from build123d import *

# Parameters (mm, degrees)
BOX697_W                     = 6
BOX697_H                     = 6
BOX697_DEPTH                 = 2
BOX697_PLACEMENT_ANGLE       = 45
BOX703_W                     = 6
BOX703_H                     = 6
BOX703_DEPTH                 = 2
BOX703_PLACEMENT_ANGLE       = 45
BOX702_W                     = 6
BOX702_H                     = 6
BOX702_DEPTH                 = 2
BOX701_W                     = 6
BOX701_H                     = 6
BOX701_DEPTH                 = 2
BOX701_PLACEMENT_ANGLE       = 225
BOX700_W                     = 6
BOX700_H                     = 6
BOX700_DEPTH                 = 2
BOX699_W                     = 6
BOX699_H                     = 6
BOX699_DEPTH                 = 2
BOX699_PLACEMENT_ANGLE       = 135
BOX698_W                     = 6
BOX698_H                     = 6
BOX698_DEPTH                 = 2
BOX696_W                     = 6
BOX696_H                     = 6
BOX696_DEPTH                 = 2
CYLINDER1770_R               = 1.5
CYLINDER1770_DEPTH           = 30
CYLINDER1770_PLACEMENT_ANGLE = 45
CYLINDER1768_R               = 1.5
CYLINDER1768_DEPTH           = 30
CYLINDER1764_R               = 1.5
CYLINDER1764_DEPTH           = 30
CYLINDER1764_PLACEMENT_ANGLE = 135
CYLINDER1767_R               = 1.5
CYLINDER1767_DEPTH           = 30
CYLINDER1765_R               = 1.5
CYLINDER1765_DEPTH           = 30
CYLINDER1765_PLACEMENT_ANGLE = 225
CYLINDER1769_R               = 1.5
CYLINDER1769_DEPTH           = 30
CYLINDER1766_R               = 1.5
CYLINDER1766_DEPTH           = 30
CYLINDER1766_PLACEMENT_ANGLE = 45
CYLINDER1771_R               = 1.5
CYLINDER1771_DEPTH           = 30
TUBE086_R                    = 35
TUBE086_R_2                  = 29.1
TUBE086_DEPTH                = 16


with BuildPart() as krychle697:
    # Box697 → Box697 (new body)
    with BuildSketch(Plane.XY):
        with Locations((3, 3)):
            Rectangle(BOX697_W, BOX697_H)
    extrude(amount=BOX697_DEPTH)


with BuildPart() as krychle697_1:
    # Box697 placement: moved
    add(krychle697.part.moved(Location((22.627417, -26.870058, 6))).rotate(Axis((22.627417, -26.870058, 6), (0, 0, 1)), BOX697_PLACEMENT_ANGLE))


with BuildPart() as krychle703:
    # Box703 → Box703 (new body)
    with BuildSketch(Plane.XY):
        with Locations((3, 3)):
            Rectangle(BOX703_W, BOX703_H)
    extrude(amount=BOX703_DEPTH)


with BuildPart() as krychle703_1:
    # Box703 placement: moved
    add(krychle703.part.moved(Location((-26.870058, -22.627417, 6))).rotate(Axis((-26.870058, -22.627417, 6), (0, 0, -1)), BOX703_PLACEMENT_ANGLE))


with BuildPart() as krychle702:
    # Box702 → Box702 (new body)
    with BuildSketch(Plane(origin=(-35, 3, 6), x_dir=(0, -1, 0), z_dir=(0, 0, 1))):
        with Locations((3, 3)):
            Rectangle(BOX702_W, BOX702_H)
    extrude(amount=BOX702_DEPTH)


with BuildPart() as krychle701:
    # Box701 → Box701 (new body)
    with BuildSketch(Plane.XY):
        with Locations((3, 3)):
            Rectangle(BOX701_W, BOX701_H)
    extrude(amount=BOX701_DEPTH)


with BuildPart() as krychle701_1:
    # Box701 placement: moved
    add(krychle701.part.moved(Location((-22.627417, 26.870058, 6))).rotate(Axis((-22.627417, 26.870058, 6), (0, 0, 1)), BOX701_PLACEMENT_ANGLE))


with BuildPart() as krychle700:
    # Box700 → Box700 (new body)
    with BuildSketch(Plane(origin=(3, 35, 6), x_dir=(-1, 0, 0), z_dir=(0, 0, 1))):
        with Locations((3, 3)):
            Rectangle(BOX700_W, BOX700_H)
    extrude(amount=BOX700_DEPTH)


with BuildPart() as krychle699:
    # Box699 → Box699 (new body)
    with BuildSketch(Plane.XY):
        with Locations((3, 3)):
            Rectangle(BOX699_W, BOX699_H)
    extrude(amount=BOX699_DEPTH)


with BuildPart() as krychle699_1:
    # Box699 placement: moved
    add(krychle699.part.moved(Location((26.870058, 22.627417, 6))).rotate(Axis((26.870058, 22.627417, 6), (0, 0, 1)), BOX699_PLACEMENT_ANGLE))


with BuildPart() as krychle698:
    # Box698 → Box698 (new body)
    with BuildSketch(Plane(origin=(35, -3, 6), x_dir=(0, 1, 0), z_dir=(0, 0, 1))):
        with Locations((3, 3)):
            Rectangle(BOX698_W, BOX698_H)
    extrude(amount=BOX698_DEPTH)


with BuildPart() as compound878:
    # Box696 → Box696 (new body)
    with BuildSketch(Plane(origin=(-3, -35, 6), x_dir=(1, 0, 0), z_dir=(0, 0, 1))):
        with Locations((3, 3)):
            Rectangle(BOX696_W, BOX696_H)
    extrude(amount=BOX696_DEPTH)

    # Compound878: union Krychle697, Krychle703, Krychle702, Krychle701, Krychle700, Krychle699, Krychle698
    add(krychle697_1.part)
    add(krychle703_1.part)
    add(krychle702.part)
    add(krychle701_1.part)
    add(krychle700.part)
    add(krychle699_1.part)
    add(krychle698.part)


with BuildPart() as obj1:
    # Cylinder1770 → Cylinder1770 (new body)
    with BuildSketch(Plane.XY):
        Circle(CYLINDER1770_R)
    extrude(amount=CYLINDER1770_DEPTH)


with BuildPart() as obj1_1:
    # Cylinder1770 placement: moved
    add(obj1.part.moved(Location((22.627417, -22.627417, 0))).rotate(Axis((22.627417, -22.627417, 0), (0, 0, 1)), CYLINDER1770_PLACEMENT_ANGLE))


with BuildPart() as obj2:
    # Cylinder1768 → Cylinder1768 (new body)
    with BuildSketch(Plane(origin=(32, 0, 0), x_dir=(0, 1, 0), z_dir=(0, 0, 1))):
        Circle(CYLINDER1768_R)
    extrude(amount=CYLINDER1768_DEPTH)


with BuildPart() as obj3:
    # Cylinder1764 → Cylinder1764 (new body)
    with BuildSketch(Plane.XY):
        Circle(CYLINDER1764_R)
    extrude(amount=CYLINDER1764_DEPTH)


with BuildPart() as obj3_1:
    # Cylinder1764 placement: moved
    add(obj3.part.moved(Location((22.627417, 22.627417, 0))).rotate(Axis((22.627417, 22.627417, 0), (0, 0, 1)), CYLINDER1764_PLACEMENT_ANGLE))


with BuildPart() as obj4:
    # Cylinder1767 → Cylinder1767 (new body)
    with BuildSketch(Plane(origin=(0, 32, 0), x_dir=(-1, 0, 0), z_dir=(0, 0, 1))):
        Circle(CYLINDER1767_R)
    extrude(amount=CYLINDER1767_DEPTH)


with BuildPart() as obj5:
    # Cylinder1765 → Cylinder1765 (new body)
    with BuildSketch(Plane.XY):
        Circle(CYLINDER1765_R)
    extrude(amount=CYLINDER1765_DEPTH)


with BuildPart() as obj5_1:
    # Cylinder1765 placement: moved
    add(obj5.part.moved(Location((-22.627417, 22.627417, 0))).rotate(Axis((-22.627417, 22.627417, 0), (0, 0, 1)), CYLINDER1765_PLACEMENT_ANGLE))


with BuildPart() as obj6:
    # Cylinder1769 → Cylinder1769 (new body)
    with BuildSketch(Plane(origin=(-32, 0, 0), x_dir=(0, -1, 0), z_dir=(0, 0, 1))):
        Circle(CYLINDER1769_R)
    extrude(amount=CYLINDER1769_DEPTH)


with BuildPart() as obj7:
    # Cylinder1766 → Cylinder1766 (new body)
    with BuildSketch(Plane.XY):
        Circle(CYLINDER1766_R)
    extrude(amount=CYLINDER1766_DEPTH)


with BuildPart() as obj7_1:
    # Cylinder1766 placement: moved
    add(obj7.part.moved(Location((-22.627417, -22.627417, 0))).rotate(Axis((-22.627417, -22.627417, 0), (0, 0, -1)), CYLINDER1766_PLACEMENT_ANGLE))


with BuildPart() as compound881:
    # Cylinder1771 → Cylinder1771 (new body)
    with BuildSketch(Plane(origin=(0, -32, 0), x_dir=(1, 0, 0), z_dir=(0, 0, 1))):
        Circle(CYLINDER1771_R)
    extrude(amount=CYLINDER1771_DEPTH)

    # Compound881: union obj1, obj2, obj3, obj4, obj5, obj6, obj7
    add(obj1_1.part)
    add(obj2.part)
    add(obj3_1.part)
    add(obj4.part)
    add(obj5_1.part)
    add(obj6.part)
    add(obj7_1.part)


with BuildPart() as cut512:
    # Tube086 → Tube086 (new body)
    with BuildSketch(Plane.XY):
        Circle(TUBE086_R)
        Circle(TUBE086_R_2, mode=Mode.SUBTRACT)
    extrude(amount=TUBE086_DEPTH)

    # Cut511: cut Compound881
    add(compound881.part, mode=Mode.SUBTRACT)

    # Cut512: cut Compound878
    add(compound878.part, mode=Mode.SUBTRACT)


solid = cut512.part
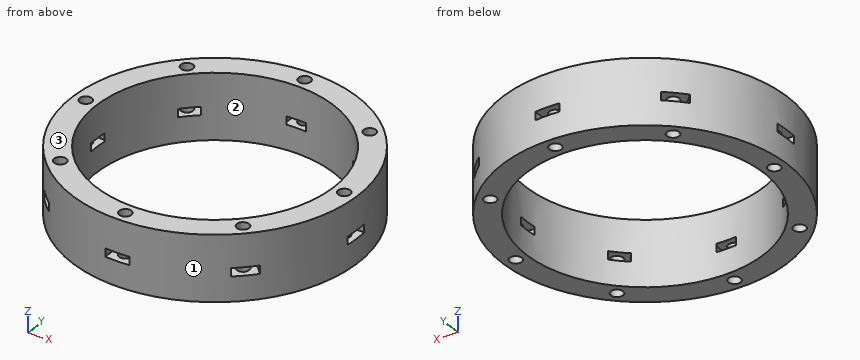
Verification items for the finished model (mm, model axes). Face numbers are marked on the shaded views. Round coordinates to 2 decimals unless told otherwise and drop trailing zeros. Order: outer loops, then holes, each group sorted by start corner. A loop starts at its lowest first (then second) coordinate and runs counter-clockwise, first axis right, second up. Notation, with made-up numbers: (65.25, 35.25) -> (118.25, 35.25) arc R22 ccw to (118.25, 48.25) -> close; hole circle Ø8 at (52, 79.5). An arc over 180 degrees is marked (long way). Put each result on its own line as item: value.
1) Section check C-C (x = 32). Record the cut outline in (y, z).
Final values:
outline: (-14.18, 0) -> (-1.5, 0) -> (-1.5, 6) -> (-3, 6) -> (-3, 8) -> (-1.5, 8) -> (-1.5, 16) -> (-14.18, 16) -> close; (1.5, 0) -> (14.18, 0) -> (14.18, 16) -> (1.5, 16) -> (1.5, 8) -> (3, 8) -> (3, 6) -> (1.5, 6) -> close
2) Depth check by flat-ended pin: pin 1 (6 mm diameter, centred on y = -25, z = 6, fed in from -X); pin 2 (1.6 mm diameter, centred on x = 32, z = 7, fed in from +Y); pin 3 (0.6 mm diameter, centred on x = 2.5, z = 6.5, fed in from +Y). Enter the tip coordinate at first touch or a pass-through.
Final values:
pin 1: stops at x = -27.22
pin 2: stops at y = 15.86
pin 3: stops at y = 29
3) Section check A-A (x = 0). Give the number of separate pieces and of enclosed holes in the cut face, then the cut area to 3 significant figures.
Final values:
separate pieces: 8
enclosed holes: 0
area: 81.2 mm^2
4) Material ranges on line 1 (Y direction, x = 0, z = 1.4); line 2 (X direction, y = 23, z = 14.5); line 3 (X direction, y = 18, z = 12.75), recorded low to high.
Final values:
line 1: y = -35 to -33.5, -30.5 to -29.1, 29.1 to 30.5, 33.5 to 35
line 2: x = -26.38 to -24.08, -21.17 to -17.83, 17.83 to 21.17, 24.08 to 26.38
line 3: x = -30.02 to -22.87, 22.87 to 30.02
5) Mould release check, pull along Y, two halves, no side actions. Record for the marked faces 1, 2 and 3: +Y half, -Y half, draft (parallel to the pull), parting line (faces both ways), or undercut.
Final values:
face 1: parting line
face 2: undercut
face 3: draft
